The listing builds one solid part. Answer for the finished solid, in the listing's coordinates (mm). A direction names the side the tool comes from. Round coordinates to 2 decimals unless told otherwise and drop trailing zeros. Write each loop counter-clockwise with the first axis right and the second up, starting at its lowest first coordinate (ties: lowest second). Pieces come first, ordered by that corner, then holes.
(1) Each of these flat-tipped pins is pushed along its axis until it touches: pin 1 Ø1.1 at (x, y) = (5.68, 4.83) entering from +Z; pin 2 Ø1.5 at (y, z) = (2.5, 3) entering from +X; pin 3 Ø0.9 at (x, z) = (4, 3) entering from +Y; pin 4 Ø2.5 at (x, z) = (9.63, 3) entering from -Y. Where does it stop, or does it pass through?
(2) A cutting plane is placed at B-B, the plane z = 3. Give the vertices of the cut face in (x, y).
(3) Find the intervals of material crossed by probe 1 along X at (y, z) = (5.25, 2.25); probe 2 along Y at (x, z) = (-1.25, 2.25); probe 3 along X at (y, z) = (-3.25, 2.75), in increasing order.
(4) The mould has two halves that part along X. Classify faces 3 (the face through (0, 1, 6)), 4 (the face through (10, 7.335, 3)), 5 (the face through (-6.133, -7.211, 3.042)): +X half, -X half, draft (parallel to the pull), parting line (faces both ways), or undercut.
(5) A cutting plane is placed at C-C, the plane x = 10.25. Give the vertices of the cut face in (y, z).
(6) A cutting plane is placed at A-A, the plane x = 0.75. Give the vertices of the cut face in (y, z), and give its area (3 significant figures).
(7) For faces 1 (the face through (4, 7.335, 3)), 2 (the face through (10.275, 5.094, 2.958)), determine the directions among +Z, -Z, +X, -X, +Y, -Y from which every point of the face is accessible in a straight line to the end or side of a thin tool.
(8) A cutting plane is placed at D-D, the plane z = 1. Give the vertices of the cut face in (x, y), and give its area (3 significant figures).
from build123d import *

# Parameters (mm, degrees)
BOSS_EXTRU_1_DEPTH      = 6
ESQUISSE5_R             = 4
ESQUISSE5_R_2           = 0.9
ENL_V_MAT_EXTRU_1_DEPTH = 18.390190711
CONG_3_R                = 10
CONG_4_R                = 3
CONG_5_R                = 1
ESQUISSE10_R            = 1.5
ENL_V_MAT_EXTRU_7_DEPTH = 3


with BuildPart() as part:
    # Esquisse2 → Boss.-Extru.1 (new body)
    with BuildSketch(Plane.XY):
        Polygon((-7.317378298, -8.665499885), (0.682621702, -6.665499885), (7.682621702, -0.665499885), (12.633955847, 10.334500115), (7.682621702, 10.334500115), (-7.317378298, 10.334500115), align=None)
    extrude(amount=BOSS_EXTRU_1_DEPTH)

    # Esquisse5 → Enlèv. mat.-Extru.1 (cut, through all)
    with BuildSketch(Plane(origin=(0, 0, 0), x_dir=(-1, 0, 0), z_dir=(0, 0, -1))):
        with Locations((2.317378298, 4.834500115)):
            Circle(ESQUISSE5_R)
        with Locations((-5.682621702, 4.834500115)):
            Circle(ESQUISSE5_R_2)
        with Locations((2.317378298, -3.165499885)):
            Circle(ESQUISSE5_R_2)
    extrude(amount=-ENL_V_MAT_EXTRU_1_DEPTH, mode=Mode.SUBTRACT)

    # Congé3
    cong_3_edges = [part.edges().sort_by_distance(p)[0] for p in [
        (7.682621702, -0.665499885, 3),
        (0.682621702, -6.665499885, 3),
    ]]
    fillet(cong_3_edges, radius=CONG_3_R)

    # Congé4
    cong_4_edges = [part.edges().sort_by_distance(p)[0] for p in [
        (-7.317378298, -8.665499885, 3),
    ]]
    fillet(cong_4_edges, radius=CONG_4_R)

    # Congé5
    cong_5_edges = [part.edges().sort_by_distance(p)[0] for p in [
        (12.633955847, 10.334500115, 3),
    ]]
    fillet(cong_5_edges, radius=CONG_5_R)

    # Esquisse10 → Enlèv. mat.-Extru.7 (cut)
    with BuildSketch(Plane(origin=(0, 10.334500115, 0), x_dir=(1, 0, 0), z_dir=(0, 1, 0))):
        with Locations(Location((3.633955847, -3, 0), (0, 0, 180))):
            Circle(ESQUISSE10_R)
        with Locations(Location((9.633955847, -3, 0), (0, 0, 180))):
            Circle(ESQUISSE10_R)
    extrude(amount=-ENL_V_MAT_EXTRU_7_DEPTH, mode=Mode.SUBTRACT)


solid = part.part
Solutions:
1. pin 1: passes through
1. pin 2: stops at x = 9.45
1. pin 3: stops at y = 7.33
1. pin 4: stops at y = 0.91
2. outline: (-7.32, -4.82) arc R3 ccw to (-3.59, -7.73) - (-1.61, -7.24) arc R10 ccw to (2.47, -5.13) - (5.99, -2.12) arc R10 ccw to (8.6, 1.37) - (12, 8.92) arc R1 ccw to (11.13, 10.33) - (11.13, 7.33) - (8.13, 7.33) - (8.13, 10.33) - (5.13, 10.33) - (5.13, 7.33) - (2.13, 7.33) - (2.13, 10.33) - (-7.32, 10.33) - close; hole circle Ø8 at (-2.32, 4.83); hole circle Ø1.8 at (-2.32, -3.17); hole circle Ø1.8 at (5.68, 4.83)
3. probe 1: x = -7.32 to -6.3, 1.66 to 4.88, 6.48 to 10.35
3. probe 2: y = -7.14 to 0.98, 8.69 to 10.33
3. probe 3: x = -7.32 to -3.21, -1.42 to 4.67
4. face 3: draft
4. face 4: undercut
4. face 5: parting line
5. outline: (5.04, 0) - (10.33, 0) - (10.33, 1.63) - (7.33, 1.63) - (7.33, 4.37) - (10.33, 4.37) - (10.33, 6) - (5.04, 6) - close
6. outline: (-6.32, 0) - (2.27, 0) - (2.27, 6) - (-6.32, 6) - close; (7.4, 0) - (10.33, 0) - (10.33, 6) - (7.4, 6) - close
6. area: 69.1 mm2
7. face 1: +Y
7. face 2: +Z, -Z, +X, -Y
8. outline: (-7.32, -4.82) arc R3 ccw to (-3.59, -7.73) - (-1.61, -7.24) arc R10 ccw to (2.47, -5.13) - (5.99, -2.12) arc R10 ccw to (8.6, 1.37) - (12, 8.92) arc R1 ccw to (11.09, 10.33) - (-7.32, 10.33) - close; hole circle Ø8 at (-2.32, 4.83); hole circle Ø1.8 at (-2.32, -3.17); hole circle Ø1.8 at (5.68, 4.83)
8. area: 209 mm2
